Build history of the part. All positions in model axes, mm. A direction names the side the tool comes from. Give positions to 0.01 mm unless a question says otherwise; leave off trailing zeros. Loops run counter-clockwise (first coordinate to the right, second up) from the corner with the lowest first, then second, coordinate; pieces in that order, holes last. Notation, with made-up numbers: M 89,33 L 120,33 A29 ccw 120,62 Z; hole C 8,16 d2. An arc over 180 degrees is marked long. Answer as a JSON object with one key per item and string values. Group by question number.
1. Slice it at A-A (z = 97). List the corners of the cut face in (x, y).
2. 3-axis set-ups, long thin cutter, end or side, ignore diameter. For faces 1 (the face through (-105, 124, 55)), 2 (the face through (80, 136, 63)), 3 (the face through (93.064, 148.32, 47.466)), 4 (the face through (-93.44, 50.55, -27.24)): which of +Z, -Z, +X, -X, +Y, -Y reach the whole face in a straight line?
3. Drop flat-ended pins along their axis: pin 1 Ø8 at (x, y) = (-93, 17) entering from +Z; pin 2 Ø20 at (x, y) = (-98.5, 21.5) entering from -Z; pin 3 Ø1 at (x, z) = (-9, 75) entering from -Y. Give the stop position or say it passes through.
4. Slice it at D-D (z = -7). List the corners of the cut face in (x, y).
5. Slice it at B-B (y = 121). List the corners of the cut face in (x, z), then the cut area to 3 significant figures.
6. Mould opens along X. For faces 5 (the face through (93, 15, 1.5)), 6 (the face through (-106.5, 165, 40)), 7 (the face through (93, 15, -40)) say: released by +X, released by -X, zero draft, split by the parting line, or undercut.
7. Slice it at C-C (x = 89.5). List the corners of the cut face in (y, z), then the cut area to 3 significant figures.
8. Drill centre lines: line 1 along X through (y, z) = (118.5, 35.5); line 2 along Y through (x, z) = (95.5, 116); line 3 along Z through (x, y) = (92, 89.5). Where is each one in solid material? Low to high. Write a range as [from, to].
from build123d import *

# Parameters (mm, degrees)
BOSS_EXTRUDE1_DEPTH   = 30
BOSS_EXTRUDE1_2_DEPTH = 30
SWEEP1_START          = -106.5
SWEEP1_DEPTH          = 26.5
SWEEP1_2_DEPTH        = 1.5
SWEEP2_START          = 80
SWEEP2_DEPTH          = 26.5
SWEEP2_START_2        = 105
SWEEP2_2_DEPTH        = 1.5
BOSS_EXTRUDE2_DEPTH   = 1.5
BOSS_EXTRUDE3_DEPTH   = 1.5
SKETCH7_W             = 213
SKETCH7_H             = 44.192821834
BOSS_EXTRUDE4_DEPTH   = 1.5
BOSS_EXTRUDE5_REACH   = 392.115
SKETCH9_W             = 222.593563538
SKETCH9_H             = 76.90916357
CUT_EXTRUDE1_DEPTH    = 487.5


# Read off the part's stored shape, not the designer's step: Sweep1, Sweep2
with BuildPart() as part:
    # Sketch1 → Boss-Extrude1 (new body)
    with BuildSketch(Plane(origin=(0, 0, 0), x_dir=(1, 0, 0), z_dir=(0, 1, 0))):
        Polygon((-80, 0), (-80, -1.5), (-106.5, -1.5), (-106.5, 42.692821834), (-80, 42.692821834), (-80, 41.192821834), (-105, 41.192821834), (-105, 0), align=None)
    extrude(amount=BOSS_EXTRUDE1_DEPTH)

    # Sweep1 outline → Sweep1 (add)
    with BuildSketch(Plane.YZ.offset(SWEEP1_START)):
        Polygon((30, -42.692821834), (270, 137.764932896), (270, 139.264932896), (30, -41.192821834), align=None)
        Polygon((30, 0), (270, 180.45775473), (270, 181.95775473), (30, 1.5), align=None)
    extrude(amount=SWEEP1_DEPTH)

    # Sweep1 2 outline → Sweep1 2 (add)
    with BuildSketch(Plane.YZ.offset(SWEEP1_START)):
        Polygon((30, -41.192821834), (270, 139.264932896), (270, 180.45775473), (30, 0), align=None)
    extrude(amount=SWEEP1_2_DEPTH)

    # Sketch5 → Boss-Extrude2 (add)
    with BuildSketch(Plane(origin=(-80, 0, 0), x_dir=(0, 0, -1), z_dir=(1, 0, 0))):
        Polygon((0, 30), (-180.45775473, 270), (-139.264932896, 270), (41.192821834, 30), align=None)
    extrude(amount=-BOSS_EXTRUDE2_DEPTH)



with BuildPart() as body_2:
    # Sketch1 → Boss-Extrude1 2 (new body)
    with BuildSketch(Plane(origin=(0, 0, 0), x_dir=(1, 0, 0), z_dir=(0, 1, 0))):
        Polygon((80, 0), (105, 0), (105, 40), (80, 40), (80, 41.5), (106.5, 41.5), (106.5, -1.5), (80, -1.5), align=None)
    extrude(amount=BOSS_EXTRUDE1_2_DEPTH)

    # Sweep2 outline → Sweep2 (add)
    with BuildSketch(Plane.YZ.offset(SWEEP2_START)):
        Polygon((270, 180.45775473), (270, 181.95775473), (30, 1.5), (30, 0), align=None)
        Polygon((270, 138.95775473), (270, 140.45775473), (30, -40), (30, -41.5), align=None)
    extrude(amount=SWEEP2_DEPTH)

    # Sweep2 2 outline → Sweep2 2 (add)
    with BuildSketch(Plane.YZ.offset(SWEEP2_START_2)):
        Polygon((270, 140.45775473), (270, 180.45775473), (30, 0), (30, -40), align=None)
    extrude(amount=SWEEP2_2_DEPTH)

    # Sketch6 → Boss-Extrude3 (add)
    with BuildSketch(Plane.ZY.offset(-80)):
        Polygon((-40, 30), (140.45775473, 270), (180.45775473, 270), (0, 30), align=None)
    extrude(amount=-BOSS_EXTRUDE3_DEPTH)


with BuildPart() as part_1:
    add(part.part)

    add(body_2.part)  # Boss-Extrude4 merges body 2
    # Sketch7 → Boss-Extrude4 (add)
    with BuildSketch(Plane(origin=(0, 270, 0), x_dir=(1, 0, 0), z_dir=(0, 1, 0))):
        with Locations((0, -159.861343813)):
            Rectangle(SKETCH7_W, SKETCH7_H)
    extrude(amount=BOSS_EXTRUDE4_DEPTH)

    # Boss-Extrude5: up to this face of the body (flat: up to its plane)
    boss_extrude5_end = Plane(part_1.part.faces().sort_by_distance((106.5, 135.770686917, 60.769229512))[0])
    # Sketch8 → Boss-Extrude5 (add, up to the picked face)
    with BuildSketch(Plane.ZY.offset(106.5), mode=Mode.PRIVATE) as boss_extrude5_sk1:
        Polygon((-11.351006958, 71.683083011), (137.764932896, 270), (137.764932896, 271.5), (138.892793863, 271.5), (66.958703747, 325.587768295), (-83.285097074, 125.770851306), align=None)
    boss_extrude5_tool1 = split(extrude(boss_extrude5_sk1.sketch, amount=-BOSS_EXTRUDE5_REACH, mode=Mode.PRIVATE), bisect_by=boss_extrude5_end, keep=Keep.BOTH, mode=Mode.PRIVATE)
    add(boss_extrude5_tool1.solids().sort_by(Axis((-106.5, 198.632705, 27.7997), (1, 0, 0)))[0])

    # Sketch9 → Cut-Extrude1 (cut)
    with BuildSketch(Plane(origin=(0, 85.429976286, -113.617695949), x_dir=(-1, 0, 0), z_dir=(0, 0.6009752032818666, -0.7992676679563107))):
        with Locations((4.796781769, 338.926878661)):
            Rectangle(SKETCH9_W, SKETCH9_H)
    extrude(amount=-CUT_EXTRUDE1_DEPTH, mode=Mode.SUBTRACT)


solid = part_1.part
Established:
{
 "1": {"outline": "M -106.5,157.01 L -80,157.01 L -80,215.78 L 106.5,215.78 L 106.5,303 L -106.5,303 Z; M 80,157.01 L 106.5,157.01 L 106.5,214.2 L 80,214.2 Z; hole M -105,159.01 L -81.5,159.01 L -81.5,213.79 L -105,213.79 Z; hole M 81.5,159.01 L 105,159.01 L 105,212.2 L 81.5,212.2 Z"},
 "2": {"face 1": "none", "face 2": "+Z, -Y", "face 3": "+X", "face 4": "-Z, +X, -X"},
 "3": {"pin 1": "stops at z = 1.5", "pin 2": "stops at z = -42.69", "pin 3": "stops at y = 185.86"},
 "4": {"outline": "M -106.5,0 L -105,0 L -105,75.47 L -81.5,75.47 L -81.5,30 L -80,30 L -80,77.47 L 106.5,77.47 L 106.5,227.23 L -106.5,227.23 Z; M 80,30 L 81.5,30 L 81.5,73.89 L 105,73.89 L 105,0 L 106.5,0 L 106.5,75.88 L 80,75.88 Z"},
 "5": {"outline": "M -106.5,-76.94 L 106.5,-76.94 L 106.5,25.73 L -80,25.73 L -80,69.92 L -106.5,69.92 Z; M 80,26.92 L 106.5,26.92 L 106.5,69.92 L 80,69.92 Z; hole M -105,27.23 L -81.5,27.23 L -81.5,68.42 L -105,68.42 Z; hole M 81.5,28.42 L 105,28.42 L 105,68.42 L 81.5,68.42 Z", "area": "22,300 mm^2"},
 "6": {"face 5": "zero draft", "face 6": "released by -X", "face 7": "undercut"},
 "7": {"outline": "M 0,-41.5 L 30,-41.5 L 270,138.96 L 270,137.76 L 71.68,-11.35 L 125.77,-83.29 L 325.59,66.96 L 270,140.89 L 270,140.46 L 30,-40 L 0,-40 Z; M 0,0 L 30,0 L 250.99,166.17 L 250.27,167.12 L 30,1.5 L 0,1.5 Z", "area": "23,300 mm^2"},
 "8": {"line 1": "x = [-106.5, -105], [-81.5, -80], [80, 81.5], [105, 106.5]", "line 2": "y = [182.28, 184.27], [237.47, 239.47], [241.05, 288.71]", "line 3": "z = [-35.05, 2.05], [3.24, 4.74], [44.74, 46.24]"}
}
